Input: part model. Units: mm. Frame: model coordinates. A direction names the side the tool comes from. Give positions to 0.01 mm unless a question says otherwise; leave off trailing zeros. Loops run counter-clockwise (first coordinate to the right, second up) from the corner with the lowest first, then second, coordinate; pieces in that order, holes last. Notation, with made-up numbers: (-19, 6.25) -> (12, 6.25) arc R6 cw to (12, 10.25) -> close; hole circle Ø11 at (-28, 58). An arc over 180 degrees is marked (long way). One line per question, with ' | ' between items.
from build123d import *

# Parameters (mm, degrees)
BOX159_W               = 0.8
BOX159_H               = 19
BOX159_DEPTH           = 0.8
BOX160_W               = 0.8
BOX160_H               = 19
BOX160_DEPTH           = 0.8
CUT083_PLACEMENT_ANGLE = 220


with BuildPart() as cubo159:
    # Box159 → Box159 (new body)
    with BuildSketch(Plane.XY):
        with Locations((0.4, 9.5)):
            Rectangle(BOX159_W, BOX159_H)
    extrude(amount=BOX159_DEPTH)


with BuildPart() as obj1:
    # Box160 → Box160 (new body)
    with BuildSketch(Plane(origin=(0.3, 0, 0.3), x_dir=(1, 0, 0), z_dir=(0, 0, 1))):
        with Locations((0.4, 9.5)):
            Rectangle(BOX160_W, BOX160_H)
    extrude(amount=BOX160_DEPTH)

    # Cut083: cut Cubo159
    add(cubo159.part, mode=Mode.SUBTRACT)


with BuildPart() as obj1_1:
    # Cut083 placement: moved
    add(obj1.part.moved(Location((-218.3, 82.4, -1.45))).rotate(Axis((-218.3, 82.4, -1.45), (0, 0, 1)), CUT083_PLACEMENT_ANGLE))


solid = obj1_1.part
1. Pin query (flat end, axial travel): P1, Ø4, axis at x = -212.5, y = 78, coming from the -Z side. Return the tip coordinate at first contact, or that it passes through.
Determined:
P1: stops at z = -0.65
2. Reachability of faces 1 (the flat face through (-212.5, 74.7, -0.65)), 2 (the flat face through (-213.122, 74.517, -0.756)) from +Z, -Z, +X, -X, +Y, -Y: full face, straight path, thin tool, end or side. Return the list, or none.
Determined:
face 1: -Z, +X, +Y | face 2: +Z, -Z, -X, -Y
3. Section query A-A (z = -0.8). Output: boundary loops of the cut face in (x, y), then the cut area to 3 significant figures.
Determined:
outline: (-219.14, 81.69) -> (-206.93, 67.14) -> (-206.7, 67.33) -> (-218.91, 81.89) -> close | area: 5.70 mm2
4. Section query B-B (x = -215). Output: boundary loops of the cut face in (y, z).
Determined:
outline: (76.76, -1.15) -> (77.22, -1.15) -> (77.22, -0.65) -> (78, -0.65) -> (78, -0.35) -> (76.76, -0.35) -> close
5. Section query C-C (y = 72.75). Output: boundary loops of the cut face in (x, z), then the cut area to 3 significant figures.
Determined:
outline: (-211.64, -1.15) -> (-211.25, -1.15) -> (-211.25, -0.65) -> (-210.59, -0.65) -> (-210.59, -0.35) -> (-211.64, -0.35) -> close | area: 0.509 mm2
6. Ray query, line 1 along X through (y, z) = (81, -1); line 2 along X through (y, z) = (73, -0.8); line 3 along Y through (x, z) = (-216.5, -0.8). Return the intervals inside material, ascending. Write a range as from..to.
Determined:
line 1: x = -218.56..-218.17 | line 2: x = -211.85..-211.46 | line 3: y = 78.54..79.01
